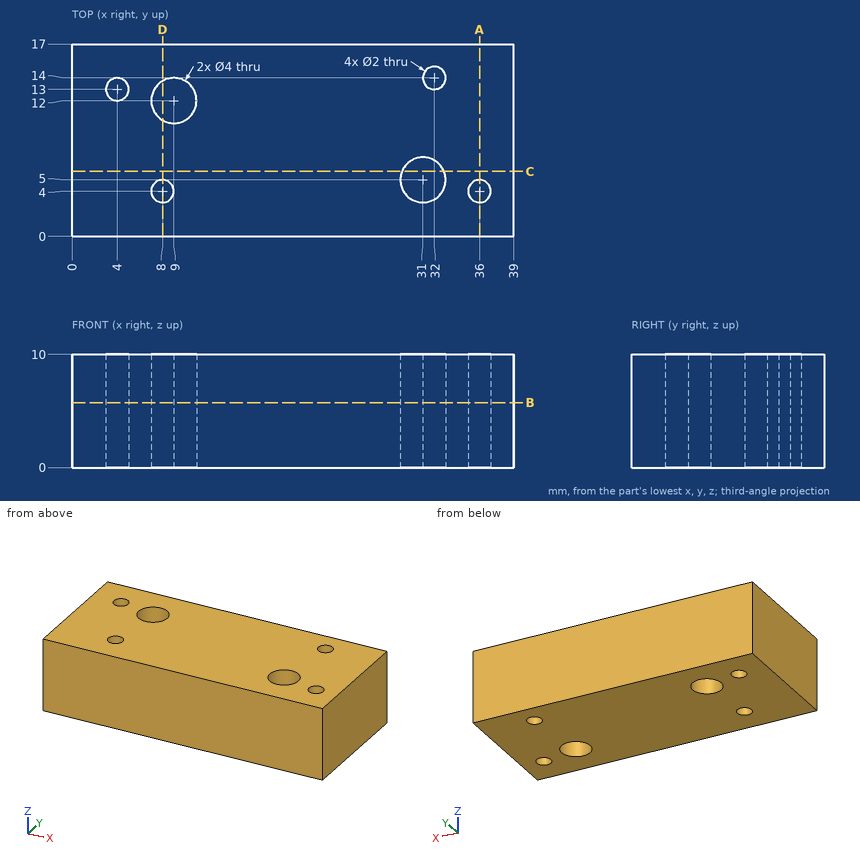
For this review, use the dimensioned drawing (mm, ordinates from the lowest corner) and the shaded views. Give positions to 0.01 mm unless a question says otherwise; leave off trailing zeros. Write each loop counter-clockwise with the first axis right and the second up, starting at its lowest first coordinate (ties: lowest second). Pieces come first, ordered by that corner, then holes.
(1) Consider section C-C, the plane y = 5.75. Give the boundary of the cut face in (x, z).
(2) Consider section D-D, the plane x = 8. Give the boundary of the cut face in (y, z), and give its area (3 significant figures).
(3) Consider section B-B, the plane z = 5.75. Give the boundary of the cut face in (x, y).
(4) To check wall thickness, follow L1, parallel to Y at x = 4, z = 3.5; L2, parallel to Y at x = 8, z = 3.5; L3, parallel to Y at x = 36, z = 5. State the ranges of each line that lie inside material, in increasing order.
(5) Consider section A-A, the plane x = 36. Give the boundary of the cut face in (y, z).
Returned:
1. outline: (0, 0) - (29.15, 0) - (29.15, 10) - (0, 10) - close; (32.85, 0) - (39, 0) - (39, 10) - (32.85, 10) - close
2. outline: (0, 0) - (3, 0) - (3, 10) - (0, 10) - close; (5, 0) - (10.27, 0) - (10.27, 10) - (5, 10) - close; (13.73, 0) - (17, 0) - (17, 10) - (13.73, 10) - close
2. area: 115 mm2
3. outline: (0, 0) - (39, 0) - (39, 17) - (0, 17) - close; hole circle Ø2 at (4, 13); hole circle Ø2 at (8, 4); hole circle Ø4 at (9, 12); hole circle Ø4 at (31, 5); hole circle Ø2 at (32, 14); hole circle Ø2 at (36, 4)
4. L1: y = 0 to 12, 14 to 17
4. L2: y = 0 to 3, 5 to 10.27, 13.73 to 17
4. L3: y = 0 to 3, 5 to 17
5. outline: (0, 0) - (3, 0) - (3, 10) - (0, 10) - close; (5, 0) - (17, 0) - (17, 10) - (5, 10) - close
